Geometry check sheet. Reference: the model listing, model coordinates, mm. A direction names the side the tool comes from. Round coordinates to 2 decimals unless told otherwise and drop trailing zeros. Write each loop counter-clockwise with the first axis right and the second up, starting at its lowest first coordinate (ties: lowest second). Pieces come first, ordered by that corner, then holes. Notation, with made-up numbers: M 82.25,73.25 L 90.25,73.25 A5 cw 90.25,78.25 Z; hole C 86,-21.75 d6. An arc over 180 degrees is marked long. Put each result on its own line as item: value. Start each with the question number.
(1) Gauge pin test, flat ends, axial feed: pin 1 (4 mm diameter, centred on x = 10.5, y = 12.5, fed in from +Z); pin 2 (1.1 mm diameter, centred on y = 24.5, z = 9.5, fed in from -X); pin 3 (0.6 mm diameter, centred on x = 9, z = 7.5, fed in from -Y); pin 4 (5 mm diameter, centred on x = 15.5, z = 9.5, fed in from +Y). Record the tip position at first contact, or that the pin passes through.
(2) Section check B-B on y = 2. Record the cut outline in (x, z), then the cut area to 3 significant figures.
(3) Section check D-D on x = -16.25. Record the cut outline in (y, z), then the cut area to 3 significant figures.
(4) Material ranges on probe 1 along Y at (x, z) = (9.85, 8); probe 2 along X at (y, z) = (27, 8); probe 3 along X at (y, z) = (21.5, 14.25), recorded low to high.
(5) Tool access check on faces 4 (the flat face through (-7.5, -4.5, 9)), 5 (the flat face through (-11, 27, 6)), 6 (the flat face through (9, 20, 5)), 7 (the flat face through (-13.5, 24.5, 9)). Record the directions out of +Z, -Z, +X, -X, +Y, -Y that give a thin tool (end or side, any length) a straight path to the whole face; none if there is none.
(6) Section check A-A on x = 9. Record the cut outline in (y, z), then the cut area to 3 significant figures.
(7) Section check C-C on x = -9.5. Record the cut outline in (y, z), then the cut area to 3 significant figures.
(8) Mould release check, pull along X, two halves, no side actions. Record for faces 1 (the flat face through (-11, -4, 9)), 2 (the flat face through (15.5, 21, 11)), 3 (the flat face through (-19.5, -7, 6)): pulls with the +X half, pulls with the -X half, needs draft (parallel to the pull), parting line crosses it, or undercut.
from build123d import *

# Parameters (mm, degrees)
BOSS_EXTRUDE1_DEPTH  = 6
SKETCH2_R            = 1.75
CUT_EXTRUDE1_DEPTH   = 41
SKETCH3_R            = 1.5
BOSS_EXTRUDE7_DEPTH  = 5.5
SKETCH4_W            = 4
SKETCH4_H            = 12
BOSS_EXTRUDE8_DEPTH  = 6
SKETCH7_W            = 6
SKETCH7_H            = 6
CUT_EXTRUDE2_DEPTH   = 40
BOSS_EXTRUDE9_DEPTH  = 6
BOSS_EXTRUDE10_DEPTH = 10
CUT_EXTRUDE3_REACH   = 41
SKETCH12_W           = 6
SKETCH12_H           = 6
BOSS_EXTRUDE11_DEPTH = 1
SKETCH13_W           = 6
SKETCH13_H           = 6
BOSS_EXTRUDE12_DEPTH = 1


with BuildPart() as part:
    # Sketch1 → Boss-Extrude1 (new body)
    with BuildSketch(Plane.XY):
        Polygon((6, 4), (-4, 4), (-4, -5), (-19.5, -5), (-19.5, -10), (0, -10), (4.75, 0), (11.5, 0), (11.5, 20), (4.75, 20), (0, 30), (-19.5, 30), (-19.5, 25), (-4, 25), (-4, 16), (6, 16), align=None)
    extrude(amount=BOSS_EXTRUDE1_DEPTH)

    # Sketch2 → Cut-Extrude1 (cut, through all)
    with BuildSketch(Plane.XZ.offset(10)):
        with Locations((9, 3)):
            Circle(SKETCH2_R)
        with Locations((-16.25, 3)):
            Circle(SKETCH2_R)
    extrude(amount=-CUT_EXTRUDE1_DEPTH, mode=Mode.SUBTRACT)

    # Sketch3 → Boss-Extrude7 (add)
    with BuildSketch(Plane(origin=(11.5, 0, 0), x_dir=(0, 0, -1), z_dir=(1, 0, 0))):
        with BuildLine():
            Line((-8, 12), (-6, 12))
            Line((-6, 12), (-6, 20))
            Line((-6, 20), (-8, 20))
            ThreePointArc((-8, 20), (-12, 16), (-8, 12))
        make_face()
        with Locations((-8, 16)):
            Circle(SKETCH3_R, mode=Mode.SUBTRACT)
    extrude(amount=-BOSS_EXTRUDE7_DEPTH)

    # Sketch4 → Boss-Extrude8 (add)
    with BuildSketch(Plane.XY.offset(6)):
        with Locations((-2, 10)):
            Rectangle(SKETCH4_W, SKETCH4_H)
        Polygon((-4, 16), (-4, 25), (-19.5, 25), (-19.5, 30), (0, 30), (0, 24), (0, 16), align=None)
        Polygon((-19.5, -5), (-19.5, -10), (0, -10), (0, 4), (-4, 4), (-4, -5), align=None)
    extrude(amount=BOSS_EXTRUDE8_DEPTH)

    # Sketch7 → Cut-Extrude2 (cut)
    with BuildSketch(Plane.XZ.offset(10)):
        with Locations((-10.5, 3)):
            Rectangle(SKETCH7_W, SKETCH7_H)
    extrude(amount=-CUT_EXTRUDE2_DEPTH, mode=Mode.SUBTRACT)

    # Sketch9 → Boss-Extrude9 (add)
    with BuildSketch(Plane(origin=(0, 0, 0), x_dir=(-1, 0, 0), z_dir=(0, 0, -1))):
        Polygon((-17.5, 17.5), (-11.5, 12), (-11.5, 20), (-13.5, 20), (-13.5, 25), (-19.5, 25), (-19.5, 20), (-19.5, 17.5), align=None)
    extrude(amount=-BOSS_EXTRUDE9_DEPTH)

    # Sketch10 → Boss-Extrude10 (add)
    with BuildSketch(Plane.XY.offset(6)):
        Polygon((19.5, 25), (15.5, 25), (15.5, 17.5), (17, 17.5), (17.5, 17.5), (19.5, 17.5), align=None)
    extrude(amount=BOSS_EXTRUDE10_DEPTH)

    # Sketch11 → Cut-Extrude3 (cut, up to next)
    with BuildSketch(Plane(origin=(19.5, 0, 0), x_dir=(0, 0, -1), z_dir=(1, 0, 0)), mode=Mode.PRIVATE) as cut_extrude3_sk1:
        with BuildLine():
            Line((-12.25, 25), (-16, 25))
            Line((-16, 25), (-16, 21.25))
            ThreePointArc((-16, 21.25), (-14.901650429, 23.901650429), (-12.25, 25))
        make_face()
    cut_extrude3_tool1 = extrude(cut_extrude3_sk1.sketch, amount=-CUT_EXTRUDE3_REACH, mode=Mode.PRIVATE) & part.part
    add(cut_extrude3_tool1.solids().sort_by_distance((19.5, 24.16237, 15.16237))[0], mode=Mode.SUBTRACT)
    # Sketch11 → Cut-Extrude3 (cut, up to next)
    with BuildSketch(Plane(origin=(19.5, 0, 0), x_dir=(0, 0, -1), z_dir=(1, 0, 0)), mode=Mode.PRIVATE) as cut_extrude3_sk2:
        with BuildLine():
            ThreePointArc((-12.25, 17.5), (-14.901650429, 18.598349571), (-16, 21.25))
            Line((-16, 21.25), (-16, 17.5))
            Line((-16, 17.5), (-12.25, 17.5))
        make_face()
    cut_extrude3_tool2 = extrude(cut_extrude3_sk2.sketch, amount=-CUT_EXTRUDE3_REACH, mode=Mode.PRIVATE) & part.part
    add(cut_extrude3_tool2.solids().sort_by_distance((19.5, 18.33763, 15.16237))[0], mode=Mode.SUBTRACT)

    # Sketch12 → Boss-Extrude11 (add)
    with BuildSketch(Plane.XZ.offset(-25)):
        with Locations((-10.5, 9)):
            Rectangle(SKETCH12_W, SKETCH12_H)
    extrude(amount=BOSS_EXTRUDE11_DEPTH)

    # Sketch13 → Boss-Extrude12 (add)
    with BuildSketch(Plane(origin=(0, -5, 0), x_dir=(1, 0, 0), z_dir=(0, 1, 0))):
        with Locations((-10.5, -9)):
            Rectangle(SKETCH13_W, SKETCH13_H)
    extrude(amount=BOSS_EXTRUDE12_DEPTH)


solid = part.part
Answers follow:
1. pin 1: stops at z = 11.71
1. pin 2: stops at x = -19.5
1. pin 3: stops at y = 12
1. pin 4: stops at y = 25
2. outline: M -4,0 L 11.5,0 L 11.5,6 L 0,6 L 0,12 L -4,12 Z; hole C 9,3 d3.5
2. area: 107 mm^2
3. outline: M -10,0 L -5,0 L -5,1.25 L -10,1.25 Z; M -10,4.75 L -5,4.75 L -5,12 L -10,12 Z; M 25,0 L 30,0 L 30,1.25 L 25,1.25 Z; M 25,4.75 L 30,4.75 L 30,12 L 25,12 Z
3. area: 85.0 mm^2
4. probe 1: y = 12 to 14.5, 17.5 to 20
4. probe 2: x = -19.5 to 0
4. probe 3: x = 15.5 to 19.5
5. face 4: +Z, -Z
5. face 5: -Z, +Y, -Y
5. face 6: +Z, -Z, +Y
5. face 7: +Z, -Z, -X
6. outline: M 0,0 L 20,0 L 20,1.25 L 0,1.25 Z; M 0,4.75 L 20,4.75 L 20,8 A4 ccw 12,8 L 12,6 L 0,6 Z; hole C 16,8 d3
6. area: 84.1 mm^2
7. outline: M -10,6 L -4,6 L -4,12 L -10,12 Z; M 24,6 L 30,6 L 30,12 L 24,12 Z
7. area: 72.0 mm^2
8. face 1: needs draft
8. face 2: undercut
8. face 3: pulls with the -X half
